Read the model definition and answer for the solid it produces. Units are mm, in the model's axes. A direction names the side the tool comes from. Coordinates: 2 decimals unless noted, no trailing zeros. Loops run counter-clockwise (first coordinate to the right, second up) from the corner with the lowest first, then second, coordinate; pieces in that order, holes last. Notation, with made-up numbers: M -40,27 L 18,27 A13 ccw 18,52 Z; hole C 15,39 d9. An arc over 180 degrees is marked long. One line per item, written item: value. Start each with the question number.
1. Consider probe 1 along Y at (x, z) = (-10, 3.1); probe 2 along X at (y, z) = (6.75, 2.55); probe 3 along X at (y, z) = (13.25, 1.8). Determine where each line is inside the solid, lowest interval first.
2. Flat-ended cylindrical pins translate along their axes: pin 1 (2 mm diameter, centred on y = 2.5, z = 2.5, fed in from +X); pin 2 (2 mm diameter, centred on y = 12.5, z = 2, fed in from +X); pin 3 (2 mm diameter, centred on x = -19, z = 1, fed in from +Y); pin 4 (2 mm diameter, centred on y = 12, z = 3, fed in from -X). Find the tip coordinate at first contact, or state that the pin passes through.
3. For faces 1 (the face through (-1, 10, 2)), 2 (the face through (-10, 9, 4)), 3 (the face through (-17.5, 12, 2)), determine the directions among +Z, -Z, +X, -X, +Y, -Y from which every point of the face is accessible in a straight line to the end or side of a thin tool.
4. The part is cut by section A-A (x = -10). Write down the section's boundary in (y, z).
5. The part is cut by section C-C (y = 5). Write down the section's boundary in (x, z), then the cut area to 3 significant figures.
6. The part is cut by section B-B (z = 0.7). Write down the section's boundary in (x, y).
7. Determine the mould class of faces 4 (the face through (-2.5, 12, 2)), 5 (the face through (-12, 5, 2)), 6 (the face through (-10, 0, 2)), 7 (the face through (-19, 10, 2)) for opening direction Y: +Y half, -Y half, draft (parallel to the pull), parting line (faces both ways), or undercut.
```python
from build123d import *

# Parameters (mm, degrees)
F0_R     = 2
F0_W     = 15
F0_H     = 4
F1_DEPTH = 4


with BuildPart() as f1:
    # F0 (on Top) → F1 (new body)
    with BuildSketch(Plane.XY):
        Polygon((-20, 0), (0, 0), (0, 10), (-2.5, 10), (-17.5, 10), (-20, 10), align=None)
        with Locations((-10, 5)):
            Circle(F0_R, mode=Mode.SUBTRACT)
        with Locations((-10, 12)):
            Rectangle(F0_W, F0_H)
    extrude(amount=F1_DEPTH)


solid = f1.part
```
Answer block:
1. probe 1: y = 0 to 3, 7 to 14
1. probe 2: x = -20 to -10.97, -9.03 to 0
1. probe 3: x = -17.5 to -2.5
2. pin 1: stops at x = 0
2. pin 2: stops at x = -2.5
2. pin 3: stops at y = 10
2. pin 4: stops at x = -17.5
3. face 1: +Z, -Z, +X, +Y
3. face 2: +Z, +X, -X, +Y, -Y
3. face 3: +Z, -Z, -X, +Y
4. outline: M 0,0 L 3,0 L 3,4 L 0,4 Z; M 7,0 L 14,0 L 14,4 L 7,4 Z
5. outline: M -20,0 L -12,0 L -12,4 L -20,4 Z; M -8,0 L 0,0 L 0,4 L -8,4 Z
5. area: 64.0 mm2
6. outline: M -20,0 L 0,0 L 0,10 L -2.5,10 L -2.5,14 L -17.5,14 L -17.5,10 L -20,10 Z; hole C -10,5 d4
7. face 4: draft
7. face 5: undercut
7. face 6: -Y half
7. face 7: +Y half
